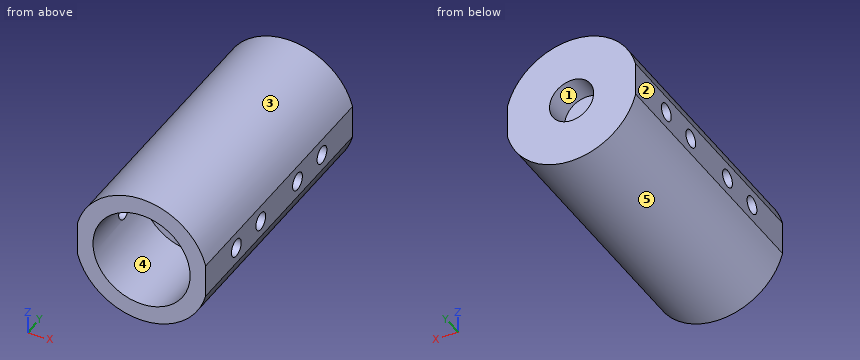
```python
from build123d import *

# Parameters (mm, degrees)
F0_R      = 19.05
F1_DEPTH  = 76.2
F2_R      = 13.97
F3_DEPTH  = 25.4
F5_DEPTH  = 76.201
F6_R      = 2.54
F7_DEPTH  = 36.8911684564
F8_R      = 6.35
F9_DEPTH  = 7.9375
F10_R     = 1.5875
F11_DEPTH = 68.2635001


with BuildPart() as f1:
    # F0 (on Front) → F1 (new body)
    with BuildSketch(Plane.XZ):
        Circle(F0_R)
    extrude(amount=F1_DEPTH)

    # F2 (on face) → F3 (cut)
    with BuildSketch(Plane.XZ.offset(76.2)):
        Circle(F2_R)
    extrude(amount=-F3_DEPTH, mode=Mode.SUBTRACT)

    # F4 (on face) → F5 (cut, through all)
    with BuildSketch(Plane.XZ.offset(76.2)):
        with BuildLine():
            ThreePointArc((18.4450827696, -4.7625016141), (19.05, -1.667e-06), (18.4450836031, 4.7624983859))
            Line((18.4450836031, 4.7624983859), (18.4450827696, -4.7625016141))
        make_face()
        with BuildLine():
            Line((-18.4450836031, -4.7624983859), (-18.4450827696, 4.7625016141))
            ThreePointArc((-18.4450827696, 4.7625016141), (-19.05, 1.667e-06), (-18.4450836031, -4.7624983859))
        make_face()
    extrude(amount=-F5_DEPTH, mode=Mode.SUBTRACT)

    # F6 (on face) → F7 (cut, through all)
    with BuildSketch(Plane(origin=(18.4450831863, 0, -1.6141e-06), x_dir=(0, 1, 0), z_dir=(1, 0, -8.75e-08))):
        with Locations((-60.325, 0)):
            Circle(F6_R)
        with Locations((-47.625, 0)):
            Circle(F6_R)
        with Locations((-28.575, 0)):
            Circle(F6_R)
        with Locations((-15.875, 0)):
            Circle(F6_R)
    extrude(amount=-F7_DEPTH, mode=Mode.SUBTRACT)

    # F8 (on face) → F9 (cut)
    with BuildSketch(Plane(origin=(0, 0, 0), x_dir=(-1, 0, 0), z_dir=(0, 1, 0))):
        Circle(F8_R)
    extrude(amount=-F9_DEPTH, mode=Mode.SUBTRACT)

    # F10 (on face) → F11 (cut, through all)
    with BuildSketch(Plane(origin=(0, -7.9375, 0), x_dir=(-1, 0, 0), z_dir=(0, 1, 0))):
        Circle(F10_R)
    extrude(amount=-F11_DEPTH, mode=Mode.SUBTRACT)


solid = f1.part
```
Work out the finished part from the listing and answer in its coordinate system (mm). Face numbers are marked on the shaded views. A direction names the side the tool comes from. Round coordinates to 2 decimals unless told otherwise and drop trailing zeros. Write each loop counter-clockwise with the first axis right and the second up, starting at its lowest first coordinate (ties: lowest second). Pieces come first, ordered by that corner, then holes. Notation, with made-up numbers: (72, 77) - (99, 77) arc R13 ccw to (99, 99) - close; hole circle Ø1 at (-37, 76.25). An arc over 180 degrees is marked (long way). Return JSON: item names as keys, results as strings. Group by question number.
Q1. The part is cut by section C-C on y = -29. Write down the section's boundary in (x, z), then the cut area to 3 significant figures.
Q2. Find the intervals of material crossed by L1, parallel to X at y = -11, z = 0; L2, parallel to Y at x = 10, z = -2; L3, parallel to X at y = -67, z = 0, in increasing order.
Q3. The mould has two halves that part along X. Classify the marked faces 1, 2 and 3: released by +X, released by -X, zero draft, split by the parting line, or undercut.
Q4. Each of these flat-tipped pins is pushed along its axis until it touches: pin 1 Ø8 at (y, z) = (-15.88, 0) entering from -X; pin 2 Ø4 at (x, z) = (0, 0) entering from -Y; pin 3 Ø3 at (y, z) = (-47.62, 0) entering from +X; pin 4 Ø4 at (x, z) = (0, 0) entering from +Y. Where does it stop, or does it pass through?
Q5. The part is cut by section D-D on x = 15. Write down the section's boundary in (y, z) (3 decimals), then the cut area to 3 significant figures.
Q6. For the marked faces 4 and 5, determine the directions among +Z, -Z, +X, -X, +Y, -Y from which every point of the face is accessible in a straight line to the end or side of a thin tool.
Solved:
{
 "1": {"outline": "(-18.45, -4.76) arc R19.05 ccw to (18.45, -4.76) - (18.45, -2.5) - (-18.45, -2.5) - close; (-18.45, 2.5) - (18.45, 2.5) - (18.45, 4.76) arc R19.05 ccw to (-18.45, 4.76) - close", "area": "948 mm²"},
 "2": {"L1": "-18.45 to -1.59, 1.59 to 18.45", "L2": "-50.8 to -49.19, -46.06 to -30.14, -27.01 to -17.44, -14.31 to 0", "L3": "-18.45 to -13.97, 13.97 to 18.45"},
 "3": {"face 1": "undercut", "face 2": "released by -X", "face 3": "split by the parting line"},
 "4": {"pin 1": "x = -18.45", "pin 2": "y = -50.8", "pin 3": "through", "pin 4": "y = -7.94"},
 "5": {"outline": "(-76.2, -11.743) - (0, -11.743) - (0, 11.743) - (-76.2, 11.743) - close; hole circle Ø5.08 at (-60.325, 0); hole circle Ø5.08 at (-47.625, 0); hole circle Ø5.08 at (-28.575, 0); hole circle Ø5.08 at (-15.875, 0)", "area": "1,710 mm²"},
 "6": {"face 4": "-Y", "face 5": "-Z, +Y, -Y"}
}
